```python
from build123d import *

# Parameters (mm, degrees)
SKETCH1_W                = 740
SKETCH1_H                = 150
BOSS_EXTRUDE1_DEPTH      = 441.94307
BOSS_EXTRUDE1_DEPTH_BACK = 198.05693
SKETCH2_W                = 620
SKETCH2_H                = 720
CUT_EXTRUDE1_DEPTH       = 150
CUT_EXTRUDE2_DEPTH       = 630


with BuildPart() as part:
    # Sketch1 → Boss-Extrude1 (new body, two sides)
    with BuildSketch(Plane(origin=(0, 0, 0), x_dir=(0, 0, -1), z_dir=(1, 0, 0))) as boss_extrude1_sk:
        with Locations((133.994417004, 1223.59608297)):
            Rectangle(SKETCH1_W, SKETCH1_H)
    extrude(amount=BOSS_EXTRUDE1_DEPTH)
    extrude(boss_extrude1_sk.sketch, amount=-BOSS_EXTRUDE1_DEPTH_BACK)

    # Sketch2 → Cut-Extrude1 (cut)
    with BuildSketch(Plane(origin=(0, 1298.59608297, 0), x_dir=(1, 0, 0), z_dir=(0, 1, 0))):
        with Locations((121.943070464, 133.994417004)):
            Rectangle(SKETCH2_W, SKETCH2_H)
    extrude(amount=-CUT_EXTRUDE1_DEPTH, mode=Mode.SUBTRACT)

    # Sketch3 → Cut-Extrude2 (cut)
    with BuildSketch(Plane(origin=(441.943070464, 0, 0), x_dir=(0, 0, -1), z_dir=(1, 0, 0))):
        Polygon((133.994417004, 1148.59608297), (333.994417004, 1148.59608297), (333.994417004, 1298.59608297), (-66.005582996, 1298.59608297), (-66.005582996, 1148.59608297), align=None)
    extrude(amount=-CUT_EXTRUDE2_DEPTH, mode=Mode.SUBTRACT)


solid = part.part
```
The listing builds one solid part. Answer for the finished solid, in the listing's coordinates (mm). A direction names the side the tool comes from. Coordinates: 2 decimals unless noted, no trailing zeros. Order: outer loops, then holes, each group sorted by start corner. A loop starts at its lowest first (then second) coordinate and runs counter-clockwise, first axis right, second up. Notation, with made-up numbers: M -25,41.5 L 10,41.5 A37 cw 10,80.5 Z; hole C 2.25,68.25 d6. An arc over 180 degrees is marked long. Answer as a JSON object with one key per item and string values. Group by question number.
1. Section A-A on z = 171.5 is taken. Write down the section's boundary in (x, y), then the cut area to 3 significant figures.
2. A tool of negligible diameter and unlimited length cuts with its end or side. For faces 1 (the flat face through (118, 1225, -493.994)), 2 (the flat face through (441.943, 1225, -418)), from which of +Z, -Z, +X, -X, +Y, -Y can it reach the whole face along a straight path? Write none if from no direction.
3. Section D-D on z = -239.5 is taken. Write down the section's boundary in (x, y), then the cut area to 3 significant figures.
4. Section C-C on y = 1187 is taken. Write down the section's boundary in (x, z).
5. Section B-B on x = 353.5 is taken. Write down the section's boundary in (y, z).
6. A flat-ended cylindrical pin translates along its axis: P1, Ø1.5, axis at y = 1198.5, z = -104, coming from the +X side. Find the tip coordinate at first contact, or state that the pin passes through.
7. Straight lines are drawn through the part: line 1 (Z direction, x = 50, y = 1276); line 2 (X direction, y = 1256.5, z = -445); line 3 (X direction, y = 1281, z = -82). For each, find the intervals that lie inside material, in ascending order.
8. Determine the mould class of faces 3 (the flat face through (126, 1223, -503.994)), 4 (the flat face through (-188.057, 1225, -129)), 5 (the flat face through (-198.057, 1225, -129)), 6 (the flat face through (126, 1223, 236.006)) for opening direction Z: released by +Z, released by -Z, zero draft, split by the parting line, or undercut.
Values follow:
{
 "1": {"outline": "M -198.06,1148.6 L -188.06,1148.6 L -188.06,1298.6 L -198.06,1298.6 Z; M 431.94,1148.6 L 441.94,1148.6 L 441.94,1298.6 L 431.94,1298.6 Z", "area": "3,000 mm2"},
 "2": {"face 1": "+Y, -Y", "face 2": "+Z, -Z, +X, +Y, -Y"},
 "3": {"outline": "M -198.06,1148.6 L -188.06,1148.6 L -188.06,1298.6 L -198.06,1298.6 Z", "area": "1,500 mm2"},
 "4": {"outline": "M -198.06,-503.99 L 441.94,-503.99 L 441.94,-333.99 L 431.94,-333.99 L 431.94,-493.99 L -188.06,-493.99 L -188.06,226.01 L 431.94,226.01 L 431.94,66.01 L 441.94,66.01 L 441.94,236.01 L -198.06,236.01 Z"},
 "5": {"outline": "M 1148.6,-503.99 L 1298.6,-503.99 L 1298.6,-493.99 L 1148.6,-493.99 Z; M 1148.6,226.01 L 1298.6,226.01 L 1298.6,236.01 L 1148.6,236.01 Z"},
 "6": {"P1": "x = -188.06"},
 "7": {"line 1": "-503.99 to -493.99, 226.01 to 236.01", "line 2": "-198.06 to -188.06, 431.94 to 441.94", "line 3": "-198.06 to -188.06"},
 "8": {"face 3": "released by -Z", "face 4": "undercut", "face 5": "zero draft", "face 6": "released by +Z"}
}
